Part print with two shaded views. Sizes in mm from the minimum x, y, z corner. Round coordinates to 2 decimals unless told otherwise and drop trailing zeros. Order: outer loops, then holes, each group sorted by start corner. A loop starts at its lowest first (then second) coordinate and runs counter-clockwise, first axis right, second up. Notation, with made-up numbers: (32, 17) - (45, 17) arc R36 ccw to (45, 51) - close; hole circle Ø11 at (71, 53.5). An arc over 180 degrees is marked (long way). Use one line per item in the form item = value.
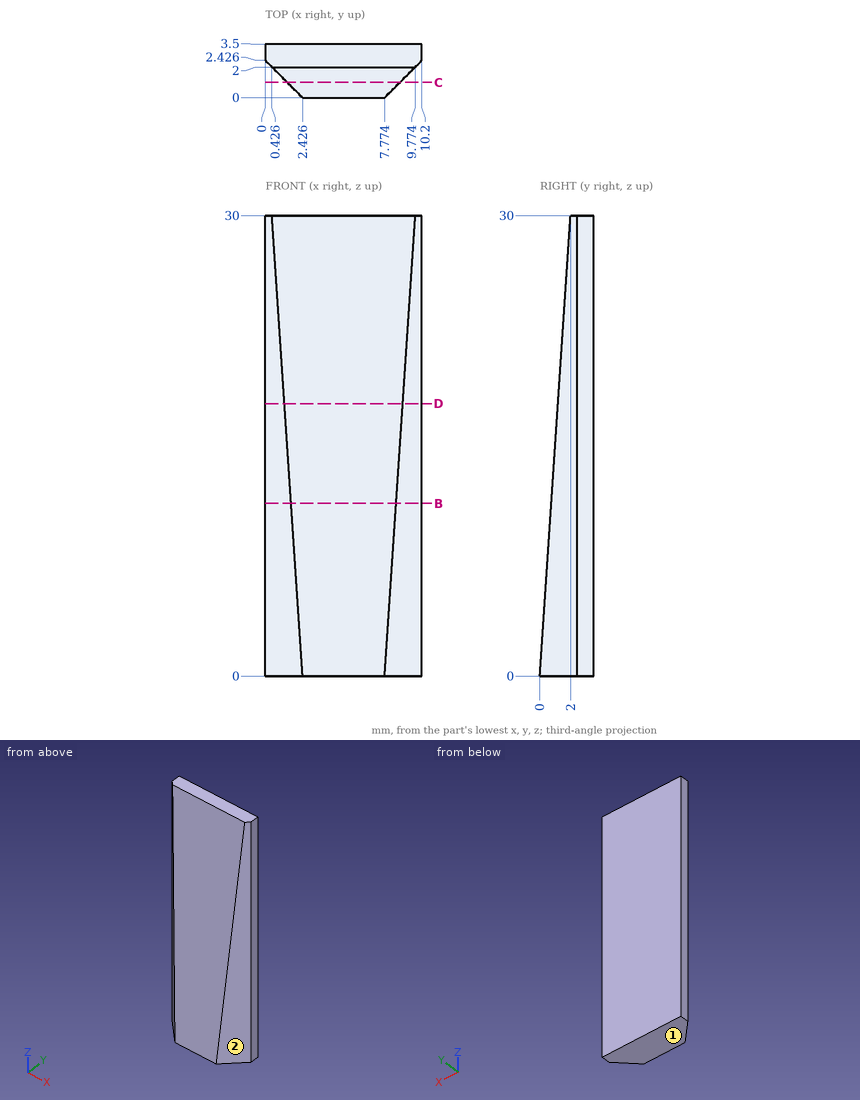
(1) Pull direction X, two halves, no side cores. Call the marked faces 1 and 2: released by +X, released by -X, zero draft, split by the parting line, or undercut.
Report:
face_1 = zero draft
face_2 = released by +X
(2) Probe probe 1 along X at (y, z) = (2, 28.5) (1 decimal); probe 2 along X at (y, z) = (2.4, 6.75) (1 decimal); probe 3 along Y at (x, z) = (4.5, 19.75). List the from-to ranges inside material, lowest first. Write a range as [from, to].
Report:
probe_1 = [0.4, 9.8]
probe_2 = [0, 10.2]
probe_3 = [1.32, 3.5]
(3) Pin check, flat tip, straight feed: pin 1 (1 mm diameter, centred on x = 1.5, z = 13, fed in from -Y). Stop position of the tip, or through.
Report:
pin_1 = 0.83
(4) Slice it at D-D on z = 17.75. Give the cut face in (x, y), then the cut area to 3 significant figures.
Report:
outline = (0, 2.43) - (1.24, 1.18) - (8.96, 1.18) - (10.2, 2.43) - (10.2, 3.5) - (0, 3.5) - close
area = 22.1 mm2
(5) Slice it at C-C on y = 1. Give the cut face in (x, z).
Report:
outline = (1.43, 0) - (8.77, 0) - (8.77, 15) - (1.43, 15) - close
(6) Slice it at B-B on z = 11.25. Give the cut face in (x, y).
Report:
outline = (0, 2.43) - (1.68, 0.75) - (8.52, 0.75) - (10.2, 2.43) - (10.2, 3.5) - (0, 3.5) - close
